```python
from build123d import *

# Parameters (mm, degrees)
SKETCH2_W           = 13
SKETCH2_H           = 5
BOSS_EXTRUDE1_DEPTH = 100
SKETCH4_W           = 46.302304271
SKETCH4_H           = 2
BOSS_EXTRUDE2_DEPTH = 10
BOSS_EXTRUDE4_DEPTH = 10


with BuildPart() as part:
    # Sketch2 → Boss-Extrude1 (new body)
    with BuildSketch(Plane(origin=(0, 5.94140841, 0), x_dir=(0, 0, -1), z_dir=(1, 0, 0))):
        Polygon((-0.588894188, 6), (4.411105812, 6), (4.411105812, 15.949875627), (-15.538894188, 15.949875627), (-15.538894188, 5.999875627), (-10.538894188, 5.999875627), (-10.538894188, 0), (-0.588894188, 0), align=None)
        Polygon((20.763410083, 14), (17.763410083, 14), (17.763410083, 0), (17.763410083, -5), (20.763410083, -5), align=None)
        Polygon((-0.588894188, 0), (4.763410083, 0), (4.763410083, -5), (-25.538894188, -5), (-25.538894188, 0), (-10.538894188, 0), align=None)
        with Locations((11.263410083, -2.5)):
            Rectangle(SKETCH2_W, SKETCH2_H)
    extrude(amount=BOSS_EXTRUDE1_DEPTH)

    # Sketch4 → Boss-Extrude2 (add)
    with BuildSketch(Plane.ZY):
        with Locations((2.387742053, 1.94140841)):
            Rectangle(SKETCH4_W, SKETCH4_H)
    extrude(amount=BOSS_EXTRUDE2_DEPTH)

    # Sketch5 → Boss-Extrude4 (add)
    with BuildSketch(Plane(origin=(100, 0, 0), x_dir=(0, 0, -1), z_dir=(1, 0, 0))):
        Polygon((-25.538894188, 5.94140841), (-25.538894188, 2.94140841), (20.763410083, 2.94140841), (20.763410083, 5.94140841), (17.763410083, 5.94140841), (-0.588894188, 5.94140841), (-10.538894188, 5.94140841), align=None)
    extrude(amount=BOSS_EXTRUDE4_DEPTH)


solid = part.part
```
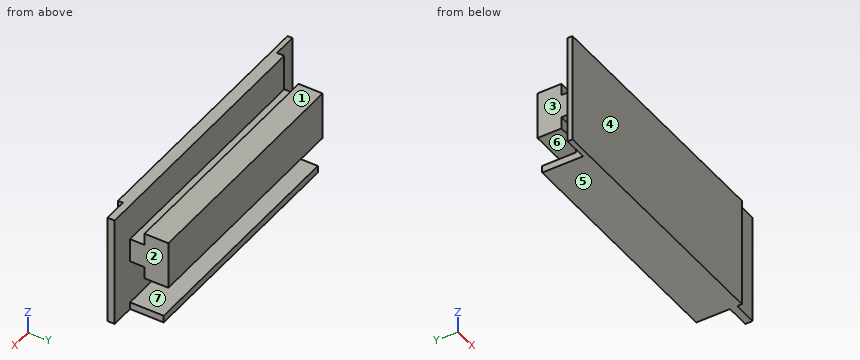
The model under review builds one solid part; all positions refer to its coordinate system, in mm. Face numbers are marked on the shaded views. A direction names the side the tool comes from. Coordinates: 2 decimals unless noted, no trailing zeros. Order: outer loops, then holes, each group sorted by start corner. A loop starts at its lowest first (then second) coordinate and runs counter-clockwise, first axis right, second up. Notation, with made-up numbers: (35.25, 89) -> (78.25, 89) arc R24 ccw to (78.25, 128) -> close; hole circle Ø1 at (-26.75, 40). An arc over 180 degrees is marked (long way). Answer in a Markdown table with one row per item. Add a question column.
Item 1: Mouldability with a two-part tool opening along Z and no side actions: class the marked faces 4, 5, 6 and 7 as +Z half, -Z half, draft (parallel to the pull), parting line (faces both ways), or undercut.
Item 2: We need section C-C on z = 5. Write out the cut boundary in (x, y).
Item 3: We need section B-B on x = 54. Write out the cut boundary in (y, z), plus the area to 3 significant figures.
Item 4: We need section A-A on y = 10. Write out the cut boundary in (x, z), plus the area to 4 significant figures.
Item 5: To check wall thickness, follow probe 1 along Z at (x, y) = (13.5, 16.75); probe 2 along Y at (x, z) = (87.5, -2); probe 3 along Z at (x, y) = (34, 6). State the ranges of each line that lie inside material, in increasing order.
Item 6: We need section D-D on y = 16.75. Write out the cut boundary in (x, z).
Item 7: Machinability: for the marked faces 1, 2 and 3, which of the approach directions +Z, -Z, +X, -X, +Y, -Y give a long, thin tool a straight path to every point of the face, cutting with its end or side? Answer none if there is none.
Item 8: Clearance check with flat-ended pins moving along their axes: pin 1 (12 mm diameter, centred on y = 13, z = -4.5, fed in from +X); pin 2 (5 mm diameter, centred on x = -3, z = 6.5, fed in from +Y); pin 3 (5 mm diameter, centred on x = 36.5, y = 10, fed in from +Z). State where each tip first meets the part, or that it passes through.
Final values:
| question | item | result |
|---|---|---|
| 1 | face 4 | draft |
| 1 | face 5 | -Z half |
| 1 | face 6 | undercut |
| 1 | face 7 | undercut |
| 2 | outline | (-10, 0.94) -> (100, 0.94) -> (100, 2.94) -> (110, 2.94) -> (110, 5.94) -> (100, 5.94) -> (100, 21.89) -> (0, 21.89) -> (0, 2.94) -> (-10, 2.94) -> close |
| 3 | outline | (0.94, -20.76) -> (19.94, -20.76) -> (19.94, -17.76) -> (5.94, -17.76) -> (5.94, 0.59) -> (11.94, 0.59) -> (11.94, -4.41) -> (21.89, -4.41) -> (21.89, 15.54) -> (11.94, 15.54) -> (11.94, 10.54) -> (5.94, 10.54) -> (5.94, 25.54) -> (0.94, 25.54) -> close |
| 3 | area | 532 mm2 |
| 4 | outline | (0, -20.76) -> (100, -20.76) -> (100, -17.76) -> (0, -17.76) -> close; (0, 0.59) -> (100, 0.59) -> (100, 10.54) -> (0, 10.54) -> close |
| 4 | area | 1,295 mm2 |
| 5 | probe 1 | z = -20.76 to -17.76, -4.41 to 15.54 |
| 5 | probe 2 | y = 0.94 to 5.94, 11.94 to 21.89 |
| 5 | probe 3 | z = -20.76 to -17.76, 0.59 to 10.54 |
| 6 | outline | (0, -20.76) -> (100, -20.76) -> (100, -17.76) -> (0, -17.76) -> close; (0, -4.41) -> (100, -4.41) -> (100, 15.54) -> (0, 15.54) -> close |
| 7 | face 1 | +Z, +X, -X, +Y |
| 7 | face 2 | +Z, -Z, +X, +Y |
| 7 | face 3 | +Z, -Z, -X, +Y |
| 8 | pin 1 | stops at x = 100 |
| 8 | pin 2 | stops at y = 2.94 |
| 8 | pin 3 | stops at z = 15.54 |
